from build123d import *

# Parameters (mm, degrees)
F0_R     = 2.5
F1_DEPTH = 10


with BuildPart() as f1:
    # F0 (on Front) → F1 (new body)
    with BuildSketch(Plane.XZ):
        Polygon((2.523419, 34.908915), (0, 40), (-2.536541, 34.907964), (-5.767684, 39.581989), (-7.530638, 34.18025), (-11.400408, 38.340979), (-12.368155, 32.74185), (-16.796091, 36.302773), (-16.948511, 30.622671), (-21.842545, 33.509748), (-21.176467, 27.866777), (-26.434842, 30.019979), (-24.964116, 24.531468), (-30.477498, 25.906025), (-28.232704, 20.686093), (-33.886457, 21.253425), (-30.914268, 16.410607), (-36.658408, 16.005034), (-33.050996, 11.516582), (-38.580196, 10.5626), (-34.308045, 6.925175), (-39.684772, 5.011874), (-34.952549, 1.821893), (-39.993003, -0.748139), (-34.859956, -3.127857), (-39.487376, -6.383347), (-34.069918, -8.015029), (-38.191725, -11.890844), (-32.598243, -12.741843), (-36.13197, -17.160441), (-30.474374, -17.213731), (-33.349323, -22.086708), (-27.740803, -21.341224), (-29.899455, -26.571086), (-24.452222, -25.041742), (-25.851387, -30.523856), (-20.674425, -28.241249), (-21.286111, -33.865934), (-16.482993, -30.875734), (-16.294963, -36.530456), (-11.961787, -32.892486), (-10.977801, -38.464112), (-7.20126, -34.251158), (-5.441006, -39.628215), (-2.296658, -34.924567), (0.204647, -39.999476), (2.653894, -34.899238), (5.846206, -39.570467), (7.551349, -34.17568), (11.3708, -38.349771), (12.297724, -32.768369), (16.667898, -36.361809), (16.798058, -30.705459), (21.631521, -33.646357), (20.962313, -28.028225), (26.162361, -30.25774), (24.707175, -24.79023), (30.169771, -26.263757), (27.95772, -21.056256), (33.573573, -21.744314), (30.648913, -16.901009), (36.305668, -16.789832), (32.726914, -12.407623), (38.311395, -11.499435), (34.150146, -7.665998), (39.550625, -5.978969), (34.890136, -2.770998), (39.998564, -0.338882), (34.932078, 2.17944), (39.646252, 5.307986), (34.275132, 7.086275), (38.500736, 10.848656), (32.948618, 11.806293), (36.584761, 16.17267), (30.908097, 16.422226), (33.878465, 21.266161), (28.224926, 20.696704), (30.467758, 25.917479), (24.954893, 24.54085), (26.423556, 30.029913), (21.16599, 27.874735), (21.829947, 33.517956), (16.936998, 30.62904), (16.782444, 36.309084), (12.355847, 32.746497), (11.385994, 38.345262), (7.517789, 34.183078), (5.752804, 39.584154), align=None)
        Circle(F0_R, mode=Mode.SUBTRACT)
    extrude(amount=F1_DEPTH)


solid = f1.part
Check sheet for the modelled part. Datum: model origin and axes. Units: mm. A direction names the side the tool comes from. Round coordinates to 2 decimals unless told otherwise and drop trailing zeros. Order: outer loops, then holes, each group sorted by start corner. A loop starts at its lowest first (then second) coordinate and runs counter-clockwise, first axis right, second up.
Q1. Draft check along X on faces 1 (the face through (4.16, -4.93, 37.28)), 2 (the face through (37.253, -4.93, -4.397)), 3 (the face through (-36.817, -4.93, -7.188)). Enter one of: pulls with the +X half, pulls with the -X half, needs draft (parallel to the pull), parting line crosses it, or undercut.
Filled sheet:
face 1: undercut
face 2: pulls with the +X half
face 3: pulls with the -X half
Q2. Scan lines: L1, parallel to Z at x = 29.5, y = -9.5; L2, parallel to Z at x = 30, y = -5.25; L3, parallel to Z at x = -2, y = -9.5. Record each from-to range of solid material in increasing order.
Filled sheet:
L1: z = -26.08 to -24.69, -21.25 to 20.83, 23.66 to 25.68
L2: z = -26.22 to -25.86, -21.31 to 20.88, 24.83 to 25.8
L3: z = -35.53 to -1.5, 1.5 to 35.99
Q3. Cross-section at B-B, the plane z = 18. Enter the section's corners in (x, y).
Filled sheet:
outline: (-31.89, -10) - (31.88, -10) - (31.88, 0) - (-31.89, 0) - close
Q4. Depth check by flat-ended pin: P1, Ø3, axis at x = 17.5, y = -6.5, coming from the -Z side; P2, Ø1.5, axis at x = 0.5, y = -6.5, coming from the -Z side; P3, Ø2, axis at x = 24, y = -4.5, coming from the +Z side; P4, Ø3, axis at x = 0, z = 0, coming from the +Y side. Enter the tip coordinate at first touch or a pass-through.
Filled sheet:
P1: stops at z = -36.36
P2: stops at z = -40
P3: stops at z = 29.45
P4: passes through
Q5. Cross-section at A-A, the plane x = 9. Enter the section's corners in (y, z), plus the area to 3 significant figures.
Filled sheet:
outline: (-10, -35.76) - (0, -35.76) - (0, 35.78) - (-10, 35.78) - close
area: 715 mm2
Q6. Set-up check for faces 4 (the face through (-27.214, -4.93, -25.817)), 5 (the face through (-35.43, -4.93, -12.31)), 6 (the face through (9.479, -4.93, 36.293)): record each of +Z, -Z, +X, -X, +Y, -Y from which the full face is reachable in a straight line by a thin tool's end or side.
Filled sheet:
face 4: +Y, -Y
face 5: -X, +Y, -Y
face 6: +Z, +Y, -Y
